The drawing under review shows one solid part. Ordinate dimensions are in mm from its lowest x, y, z. A direction names the side the tool comes from. Round coordinates to 2 decimals unless told otherwise and drop trailing zeros. Order: outer loops, then holes, each group sorted by start corner. A loop starts at its lowest first (then second) coordinate and runs counter-clockwise, first axis right, second up. Notation, with made-up numbers: M 88.5,28 L 107.5,28 A20 ccw 107.5,63 Z; hole C 14,-16 d4. An arc over 180 degrees is marked long. Answer as a JSON object with one key per item and string values. Group by question number.
1) Consider section C-C, the plane z = 8.5. Write out the cut boundary in (x, y).
2) Consider section D-D, the plane x = 14.25. Write out the cut boundary in (y, z) (1 decimal).
3) Insertion check: pin 1 Ø2 at (x, z) = (17, 10.5) entering from +Y; pin 2 Ø6 at (x, y) = (11.5, 12) entering from -Z; pin 3 Ø6 at (x, z) = (17, 9) entering from -Y; pin 4 Ø2.5 at (x, z) = (3.5, 9.24) entering from +Y (3 decimals). Each pin has a flat end and moves straight along its axis. Give the tip position at first contact, or say it passes through.
4) The part is to be moulded in two halves that separate along Y. For the marked faces 4, 5 and 6, say which applies: +Y half, -Y half, draft (parallel to the pull), parting line (faces both ways), or undercut.
5) Consider section B-B, the plane y = 9.75. Write out the cut boundary in (x, z) (1 decimal).
6) For the marked faces 1, 2 and 3, list the 3-axis set-ups (+Z, -Z, +X, -X, +Y, -Y) from which the entire face can be reached by the end or side of a thin tool; tool diameter is ignored.
7) Consider section A-A, the plane x = 3.5. Write out the cut boundary in (y, z) (1 decimal).
8) To check wall thickness, follow line 1 (Y direction, x = 1.5, z = 7); line 2 (Y direction, x = 17.75, z = 13.5) (1 decimal); line 3 (X direction, y = 15.25, z = 12.25). State the ranges of each line that lie inside material, in increasing order.
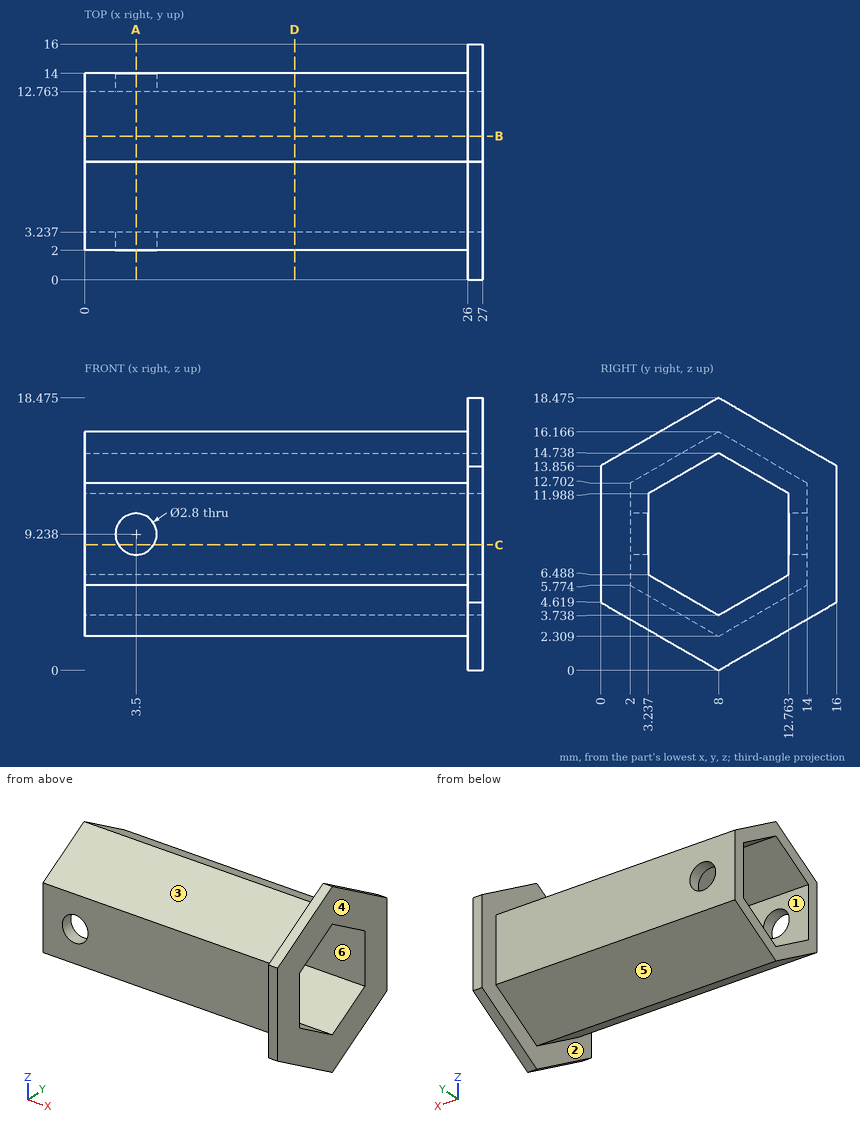
Results list:
{
 "1": {"outline": "M 0,2 L 2.31,2 L 2.31,3.24 L 0,3.24 Z; M 0,12.76 L 2.31,12.76 L 2.31,14 L 0,14 Z; M 4.69,2 L 26,2 L 26,0 L 27,0 L 27,3.24 L 4.69,3.24 Z; M 4.69,12.76 L 27,12.76 L 27,16 L 26,16 L 26,14 L 4.69,14 Z"},
 "2": {"outline": "M 2,5.8 L 8,2.3 L 14,5.8 L 14,12.7 L 8,16.2 L 2,12.7 Z; hole M 3.2,6.5 L 8,3.7 L 12.8,6.5 L 12.8,12 L 8,14.7 L 3.2,12 Z"},
 "3": {"pin 1": "y = 14", "pin 2": "z = 2.89", "pin 3": "y = 2", "pin 4": "through"},
 "4": {"face 4": "draft", "face 5": "+Y half", "face 6": "undercut"},
 "5": {"outline": "M 0,3.3 L 26,3.3 L 26,1 L 27,1 L 27,4.7 L 0,4.7 Z; M 0,13.7 L 27,13.7 L 27,17.5 L 26,17.5 L 26,15.2 L 0,15.2 Z"},
 "6": {"face 1": "+X, -X", "face 2": "-X", "face 3": "+Z, -X, -Y"},
 "7": {"outline": "M 2,5.8 L 8,2.3 L 14,5.8 L 14,7.8 L 12.8,7.8 L 12.8,6.5 L 8,3.7 L 3.2,6.5 L 3.2,7.8 L 2,7.8 Z; M 2,10.6 L 3.2,10.6 L 3.2,12 L 8,14.7 L 12.8,12 L 12.8,10.6 L 14,10.6 L 14,12.7 L 8,16.2 L 2,12.7 Z"},
 "8": {"line 1": "2 to 3.24, 12.76 to 14", "line 2": "3.4 to 5.9, 10.1 to 12.6", "line 3": "26 to 27"}
}
